Could you check a few things on this drawing? It's one solid part, dimensions in mm from its lowest x, y, z. A direction names the side the tool comes from. Give positions to 0.01 mm unless a question says otherwise; leave off trailing zeros. Order: outer loops, then holes, each group sorted by start corner. A loop starts at its lowest first (then second) coordinate and runs counter-clockwise, first axis right, second up.
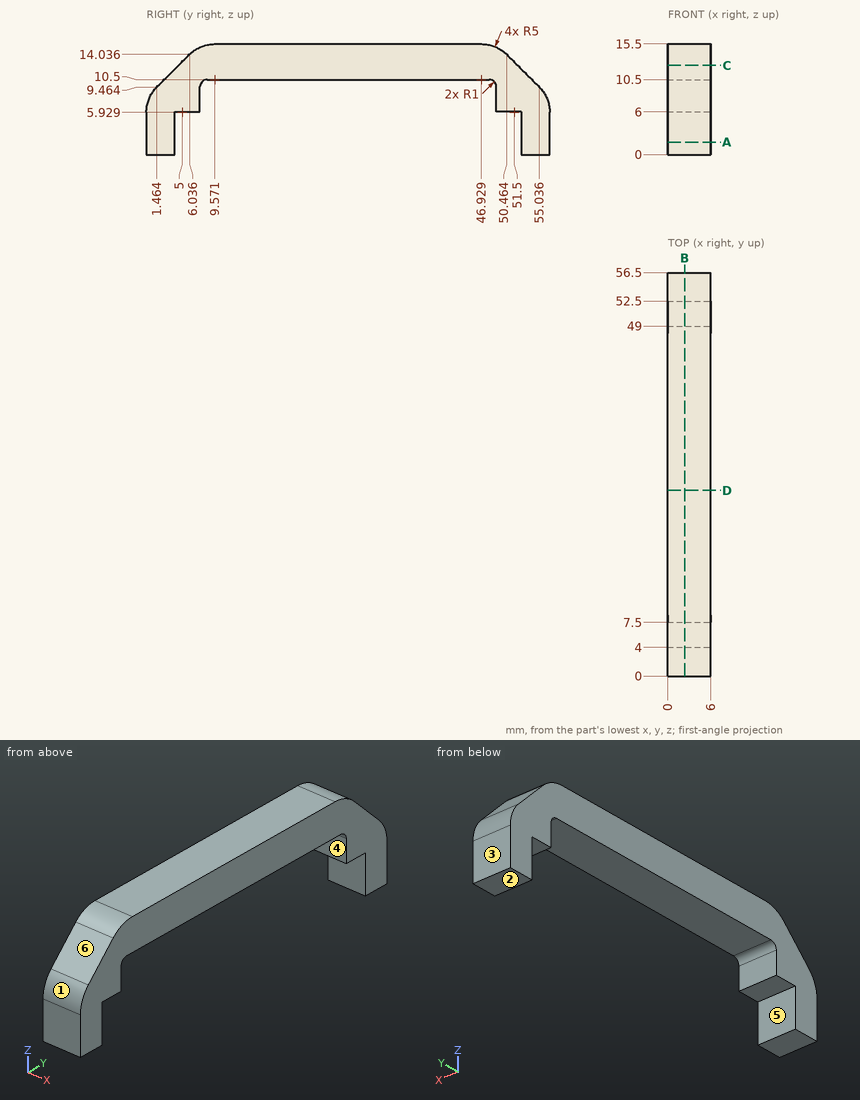
Q1. Thinking about a two-plate mould opening in Y: for the marked faces 1, 2, 3 and 4, which applies, released by +Y, released by -Y, zero draft, split by the parting line, or undercut?
Filled sheet:
face 1: released by -Y
face 2: zero draft
face 3: released by +Y
face 4: undercut
Q2. If we section it at D-D on y = 26: List the corners of the cut face in (x, z) for me.
Filled sheet:
outline: (0, 10.5) - (6, 10.5) - (6, 15.5) - (0, 15.5) - close
Q3. If we section it at C-C on z = 12.5: List the corners of the cut face in (x, y) for me.
Filled sheet:
outline: (0, 4.5) - (6, 4.5) - (6, 52) - (0, 52) - close
Q4. I'm going to push flat-ended pins straight in: P1, Ø1.5, axis at x = 4.5, y = 39, coming from the -Z side; P2, Ø1.8, axis at x = 1.5, y = 6, coming from the -Z side; P3, Ø1.8, axis at x = 2.5, z = 7.5, coming from the +Y side (1 decimal). Where does each tip first touch, or does it pass through?
Filled sheet:
P1: stops at z = 10.5
P2: stops at z = 6
P3: stops at y = 56.5
Q5. I need wall thicknesses on L1, parallel to Y at x = 3.9, z = 3; L2, parallel to Y at x = 2.9, z = 6.25; L3, parallel to Z at x = 2.25, y = 32.5. Which ranges of each line are inside material? Lowest first, please.
Filled sheet:
L1: y = 0 to 4, 52.5 to 56.5
L2: y = 0.01 to 7.5, 49 to 56.49
L3: z = 10.5 to 15.5
Q6. If we section it at A-A on z = 1.75: List the corners of the cut face in (x, y) for me.
Filled sheet:
outline: (0, 0) - (6, 0) - (6, 4) - (0, 4) - close; (0, 52.5) - (6, 52.5) - (6, 56.5) - (0, 56.5) - close
Q7. For the marked faces 5 and 6, which set-ups out of +Z, -Z, +X, -X, +Y, -Y let a thin tool reach every point of the face, with its end or its side?
Filled sheet:
face 5: -Z, +X, -X
face 6: +Z, +X, -X, -Y
Q8. If we section it at B-B on x = 2.35: List the corners of the cut face in (y, z) for me (1 decimal).
Filled sheet:
outline: (0, 0) - (4, 0) - (4, 6) - (7.5, 6) - (7.5, 9.5) arc R1 cw to (8.5, 10.5) - (48, 10.5) arc R1 cw to (49, 9.5) - (49, 6) - (52.5, 6) - (52.5, 0) - (56.5, 0) - (56.5, 5.9) arc R5 ccw to (55, 9.5) - (50.5, 14) arc R5 ccw to (46.9, 15.5) - (9.6, 15.5) arc R5 ccw to (6, 14) - (1.5, 9.5) arc R5 ccw to (0, 5.9) - close
